```python
from build123d import *

# Parameters (mm, degrees)
SKETCH1_W           = 245
SKETCH1_H           = 175
BOSS_EXTRUDE1_DEPTH = 3
SKETCH2_W           = 30
SKETCH2_H           = 2
SKETCH2_W_2         = 70.850822781
SKETCH2_H_2         = 20.149065526
SKETCH2_W_3         = 88.999828845
SKETCH2_W_4         = 16.284036158
SKETCH2_H_3         = 20
SKETCH2_W_5         = 35.753967601
SKETCH2_W_6         = 15
SKETCH2_H_4         = 15
SKETCH2_R           = 10
CUT_EXTRUDE1_DEPTH  = 151.570581456
FILLET1_R           = 25
SKETCH2_4_W         = 35.753967601
SKETCH2_4_H         = 20
SKETCH2_4_W_2       = 15
SKETCH2_4_H_2       = 15
SKETCH2_4_W_3       = 38.395009933
SKETCH2_4_H_3       = 2
SKETCH2_4_W_4       = 75
SKETCH2_4_H_4       = 10
SKETCH2_4_W_5       = 89
SKETCH2_4_W_6       = 50
SKETCH2_4_H_5       = 10.149065526
CUT_EXTRUDE2_DEPTH  = 10
SKETCH2_5_W         = 16.284036158
SKETCH2_5_H         = 20
CUT_EXTRUDE3_DEPTH  = 10
CUT_EXTRUDE4_DEPTH  = 10
CUT_EXTRUDE5_DEPTH  = 10


with BuildPart() as part:
    # Sketch1 → Boss-Extrude1 (new body)
    with BuildSketch(Plane.XY):
        Rectangle(SKETCH1_W, SKETCH1_H)
    extrude(amount=BOSS_EXTRUDE1_DEPTH)

    # Sketch2 → Cut-Extrude1 (cut, through all)
    with BuildSketch(Plane.XY.offset(3)):
        with Locations((-37.857152872, 36.074532763)):
            Rectangle(SKETCH2_W, SKETCH2_H)
        with Locations((-67.857152873, 0)):
            Rectangle(SKETCH2_W_2, SKETCH2_H_2)
        with Locations((-67.857152873, 21.074532763)):
            Rectangle(SKETCH2_W_3, SKETCH2_H)
        with Locations((-97.857152872, 36.074532763)):
            Rectangle(SKETCH2_W, SKETCH2_H)
        with Locations((-67.857152872, 56.074532763)):
            Rectangle(SKETCH2_W, SKETCH2_H)
        with Locations((0, 71.241154444)):
            Rectangle(SKETCH2_W_4, SKETCH2_H_3)
        with Locations((-33.197326406, 71.241154444)):
            Rectangle(SKETCH2_W_5, SKETCH2_H_3)
        with Locations((-67.857152872, 68.74)):
            Rectangle(SKETCH2_W_6, SKETCH2_H_4)
        Polygon((-110.669619636, 79.049728312), (-113.412388394, 75.188417537), (-102.577806523, 67.449430486), (-97.092269008, 75.172052036), (-107.926850879, 82.911039086), align=None)
        Polygon((-110.669619636, -79.049728312), (-107.926850879, -82.911039086), (-97.092269008, -75.172052036), (-102.577806523, -67.449430486), (-113.412388394, -75.188417537), align=None)
        with Locations((-67.857152872, -68.74)):
            Rectangle(SKETCH2_W_6, SKETCH2_H_4)
        with Locations((-33.197326406, -71.241154444)):
            Rectangle(SKETCH2_W_5, SKETCH2_H_3)
        with Locations((-67.857152872, -56.074532763)):
            Rectangle(SKETCH2_W, SKETCH2_H)
        with Locations((-97.857152872, -36.074532763)):
            Rectangle(SKETCH2_W, SKETCH2_H)
        with Locations((-37.857152872, -36.074532763)):
            Rectangle(SKETCH2_W, SKETCH2_H)
        with Locations((-67.857152873, -21.074532763)):
            Rectangle(SKETCH2_W_3, SKETCH2_H)
        Circle(SKETCH2_R)
    extrude(amount=-CUT_EXTRUDE1_DEPTH, mode=Mode.SUBTRACT)

    # Fillet1
    fillet1_edges = [part.edges().sort_by_distance(p)[0] for p in [
        (122.5, -87.5, 1.5),
        (-122.5, -87.5, 1.5),
        (-122.5, 87.5, 1.5),
        (122.5, 87.5, 1.5),
    ]]
    fillet(fillet1_edges, radius=FILLET1_R)

    # Sketch2_4 → Cut-Extrude2 (cut)
    with BuildSketch(Plane.XY.offset(3)):
        with Locations((33.197326406, 71.241154444)):
            Rectangle(SKETCH2_4_W, SKETCH2_4_H)
        with Locations((67.857152872, 68.74)):
            Rectangle(SKETCH2_4_W_2, SKETCH2_4_H_2)
        Polygon((113.412388394, 75.188417537), (102.577806523, 67.449430486), (97.092269008, 75.172052036), (107.926850879, 82.911039086), align=None)
        with Locations((77.104345869, 55.074532763)):
            Rectangle(SKETCH2_4_W_3, SKETCH2_4_H_3)
        with Locations((65.002938646, 32.074532763)):
            Rectangle(SKETCH2_4_W_4, SKETCH2_4_H_4)
        with Locations((72.091101618, 21.074532763)):
            Rectangle(SKETCH2_4_W_5, SKETCH2_4_H_3)
        with Locations((52.502938646, 0)):
            Rectangle(SKETCH2_4_W_6, SKETCH2_4_H_5)
        with Locations((72.091101618, -21.074532763)):
            Rectangle(SKETCH2_4_W_5, SKETCH2_4_H_3)
        with Locations((65.002938646, -32.074532763)):
            Rectangle(SKETCH2_4_W_4, SKETCH2_4_H_4)
        with Locations((72.091101618, -43.074532763)):
            Rectangle(SKETCH2_4_W_5, SKETCH2_4_H_3)
        with Locations((33.197326406, -71.241154444)):
            Rectangle(SKETCH2_4_W, SKETCH2_4_H)
        with Locations((67.857152872, -68.74)):
            Rectangle(SKETCH2_4_W_2, SKETCH2_4_H_2)
        Polygon((113.412388394, -75.188417537), (102.577806523, -67.449430486), (97.092269008, -75.172052036), (107.926850879, -82.911039086), align=None)
        with Locations((72.091101618, 43.074532763)):
            Rectangle(SKETCH2_4_W_5, SKETCH2_4_H_3)
        with Locations((77.104345869, -55.074532763)):
            Rectangle(SKETCH2_4_W_3, SKETCH2_4_H_3)
    extrude(amount=-CUT_EXTRUDE2_DEPTH, mode=Mode.SUBTRACT)

    # Sketch2_5 → Cut-Extrude3 (cut)
    with BuildSketch(Plane.XY.offset(3)):
        with Locations((0, -71.241154444)):
            Rectangle(SKETCH2_5_W, SKETCH2_5_H)
    extrude(amount=-CUT_EXTRUDE3_DEPTH, mode=Mode.SUBTRACT)

    # Sketch2_6 → Cut-Extrude4 (cut)
    with BuildSketch(Plane.XY.offset(3)):
        Polygon((5.074532763, 18.404236844), (-5.074532763, 18.404236844), (0, 13.32970408), align=None)
        Polygon((-18.404236844, -5.074532763), (-13.32970408, 0), (-18.404236844, 5.074532763), align=None)
        Polygon((-5.074532763, -18.404236844), (5.074532763, -18.404236844), (0, -13.32970408), align=None)
        Polygon((18.404236844, -5.074532763), (18.404236844, 5.074532763), (13.32970408, 0), align=None)
    extrude(amount=-CUT_EXTRUDE4_DEPTH, mode=Mode.SUBTRACT)

    # Sketch2_7 → Cut-Extrude5 (cut)
    with BuildSketch(Plane.XY.offset(3)):
        Polygon((14.127310492, -11.503503759), (15.95504041, -9.124553707), (19.919957162, -12.170770236), (18.092227245, -14.549720288), align=None)
        Polygon((18.092227245, 14.549720288), (14.127310492, 11.503503759), (15.95504041, 9.124553707), (19.919957162, 12.170770236), align=None)
        Polygon((-18.092227245, 14.549720288), (-14.127310492, 11.503503759), (-15.95504041, 9.124553707), (-19.919957162, 12.170770236), align=None)
        Polygon((-18.092227245, -14.549720288), (-14.127310492, -11.503503759), (-15.95504041, -9.124553707), (-19.919957162, -12.170770236), align=None)
    extrude(amount=-CUT_EXTRUDE5_DEPTH, mode=Mode.SUBTRACT)


solid = part.part
```
Model file for the job. Use its own axes, mm. A direction names the side the tool comes from. Coordinates: 2 decimals unless noted, no trailing zeros. Answer as a JSON object with one key per item and string values. Group by question number.
(1) Tool access for faces 4 (the face through (-2, 21, 3)), 5 (the face through (99.87, -71.26, 1.52)): list every direction of +Z, -Z, +X, -X, +Y, -Y with a clear straight run to the whole face (end or side of a thin tool).
(2) Probe line 1 along X through (y, z) = (-21, 1.3); line 2 along Y through (x, z) = (-90, 2.65); line 3 along Y through (x, z) = (20, 1.3). List the from-to ranges inside material, lowest first.
(3) Two-plate mould, pull along X, no slides. Class faces 1 (the face through (102.434, -78.987, 1.521)), 2 (the face through (-115.371, -79.982, 1.521)), 3 (the face through (114.982, -80.371, 1.521)): released by +X, released by -X, zero draft, split by the parting line, or undercut.
(4) Cut at A-A (z = 1.9). State how many separate pieces and enclosed holes the cut face has, then the cut area to 3 significant figures.
Geometry says:
{
 "1": {"face 4": "+Z, +X, -X, +Y, -Y", "face 5": "+Z, -Z"},
 "2": {"line 1": "x = -122.5 to -112.36, -23.36 to 27.59, 116.59 to 122.5", "line 2": "y = -87.5 to -37.07, -35.07 to -22.07, -20.07 to -10.07, 10.07 to 20.07, 22.07 to 35.07, 37.07 to 87.5", "line 3": "y = -87.5 to -81.24, -61.24 to 61.24, 81.24 to 87.5"},
 "3": {"face 1": "undercut", "face 2": "released by -X", "face 3": "released by +X"},
 "4": {"separate pieces": "1", "enclosed holes": "41", "area": "31,900 mm^2"}
}
